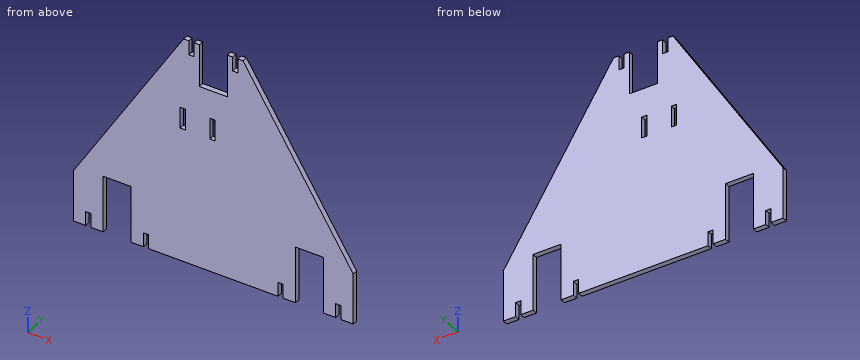
```python
from build123d import *

# Parameters (mm, degrees)
BOSS_EXTRUDE1_DEPTH = 4.7625
SKETCH2_W           = 4.7625
SKETCH2_H           = 19.05
CUT_EXTRUDE1_DEPTH  = 163.709069834


with BuildPart() as part:
    # Sketch1 → Boss-Extrude1 (new body)
    with BuildSketch(Plane(origin=(0, 0, 0), x_dir=(1, 0, 0), z_dir=(0, 1, 0))):
        Polygon((12.7, -63.5), (-12.7, -63.5), (-12.7, -101.6), (-17.4625, -101.6), (-17.4625, -88.9), (-22.225, -88.9), (-22.225, -101.6), (-26.9875, -101.6), (-127, 55.88), (-127, 101.6), (-115.8875, 101.6), (-115.8875, 88.9), (-111.125, 88.9), (-111.125, 101.6), (-100.0125, 101.6), (-100.0125, 50.8), (-74.6125, 50.8), (-74.6125, 101.6), (-63.5, 101.6), (-63.5, 88.9), (-58.7375, 88.9), (-58.7375, 101.6), (58.7375, 101.6), (58.7375, 88.9), (63.5, 88.9), (63.5, 101.6), (74.6125, 101.6), (74.6125, 50.8), (100.0125, 50.8), (100.0125, 101.6), (111.125, 101.6), (111.125, 88.9), (115.8875, 88.9), (115.8875, 101.6), (127, 101.6), (127, 55.88), (26.9875, -101.6), (22.225, -101.6), (22.225, -88.9), (17.4625, -88.9), (17.4625, -101.6), (12.7, -101.6), align=None)
    extrude(amount=BOSS_EXTRUDE1_DEPTH)

    # Sketch2 → Cut-Extrude1 (cut, through all)
    with BuildSketch(Plane(origin=(0, 4.7625, 0), x_dir=(1, 0, 0), z_dir=(0, 1, 0))):
        with Locations((-27.78125, -28.575)):
            Rectangle(SKETCH2_W, SKETCH2_H)
        with Locations((-0.79375, -28.575)):
            Rectangle(SKETCH2_W, SKETCH2_H)
    extrude(amount=-CUT_EXTRUDE1_DEPTH, mode=Mode.SUBTRACT)


solid = part.part
```
Input: part model. Units: mm. Frame: model coordinates. Round coordinates to 2 decimals unless told otherwise and drop trailing zeros. Write each loop counter-clockwise with the first axis right and the second up, starting at its lowest first coordinate (ties: lowest second). Pieces come first, ordered by that corner, then holes. Notation, with made-up numbers: M -9,-27.75 L 39,-27.75 A15 ccw 39,-0.75 Z; hole C 35,-10 d2. An arc over 180 degrees is marked long. Write each question's results on one line, items separated by ' | '.
Q1. Section query C-C (z = 35). Return loops of the section in (x, y) (1 decimal).
Results:
outline: M -69.3,0 L -30.2,0 L -30.2,4.8 L -69.3,4.8 Z; M -25.4,0 L -3.2,0 L -3.2,4.8 L -25.4,4.8 Z; M 1.6,0 L 69.3,0 L 69.3,4.8 L 1.6,4.8 Z
Q2. Line query: line 1 along X through (y, z) = (4.2, -58); line 2 along X through (y, z) = (1.95, 86.5); line 3 along X through (y, z) = (1.2, 26) (1 decimal). Output: solid intervals per line, ascending.
Results:
line 1: x = -127 to -100.01, -74.61 to 74.61, 100.01 to 127 | line 2: x = -36.58 to -12.7, 12.7 to 36.58 | line 3: x = -75 to -30.2, -25.4 to -3.2, 1.6 to 75
Q3. Section query A-A (z = -64). Return loops of the section in (x, y), and give its area (3 significant figures).
Results:
outline: M -127,0 L -100.01,0 L -100.01,4.76 L -127,4.76 Z; M -74.61,0 L 74.61,0 L 74.61,4.76 L -74.61,4.76 Z; M 100.01,0 L 127,0 L 127,4.76 L 100.01,4.76 Z | area: 968 mm^2
Q4. Pin query (flat end, axial travel): P1, Ø1.5, axis at y = 3.5, z = -54, coming from the +X side; P2, Ø2.5, axis at y = 2.5, z = 98, coming from the +X side; P3, Ø1.4, axis at y = 2, z = 29.5, coming from the -X side. Return the tip coordinate at first contact, or that it passes through.
Results:
P1: stops at x = 126.28 | P2: stops at x = 30.07 | P3: stops at x = -73.22
Q5. Section query B-B (y = 2.75). State how many separate pieces and enclosed holes the cut face has, and give its area (3 significant figures).
Results:
separate pieces: 1 | enclosed holes: 2 | area: 31,800 mm^2
Q6. Section query D-D (x = 71). Return loops of the section in (y, z).
Results:
outline: M 0,-101.6 L 4.76,-101.6 L 4.76,32.3 L 0,32.3 Z
